Source: CAD feature listing. Evaluate the final solid. Frame: model axes, mm. A direction names the side the tool comes from. Round coordinates to 2 decimals unless told otherwise and drop trailing zeros. Write each loop counter-clockwise with the first axis right and the second up, starting at its lowest first coordinate (ties: lowest second). Pieces come first, ordered by that corner, then holes. Notation, with made-up numbers: M 17,-17.5 L 29,-17.5 A5 cw 29,-12.5 Z; hole C 42,43 d8. An arc over 180 degrees is marked long. Answer in a Markdown table with one row per item. Add a question column.
Item 1: Mould query, pull axis Z, two halves, no side actions, for faces 1 (the face through (84.3, -5, 0)), 2 (the face through (94, 2, -10)), 3 (the face through (92.6, 0.1, 9)). Classes: released by +Z, released by -Z, zero draft, split by the parting line, or undercut.
Item 2: Material intervals for probe 1 along Z at (x, y) = (2, -1.1); probe 2 along Y at (x, z) = (95, -9.55); probe 3 along X at (y, z) = (1.3, 0), sorted ascending.
Item 3: Contact query for flat-ended pins moving along their axis: pin 1 (1.5 mm diameter, centred on y = 2, z = 0.5, fed in from +X); pin 2 (0.6 mm diameter, centred on y = -0.5, z = 0, fed in from -X); pin 3 (1.8 mm diameter, centred on x = 2.5, z = 0, fed in from +Y). Output: stop coordinate, or through.
Item 4: Set-up query: faces 4 (the face through (41.41, -1.5, -0.07)), 5 (the face through (2.5, -1, -0.5)), 6 (the face through (85, 0, 0)). Return all of +Z, -Z, +X, -X, +Y, -Y with unobstructed straight access to the full face (end or side cutting, diameter ignored); none if empty.
Item 5: Cut plane B-B on y = 0. Return loops of the section in (x, z).
Item 6: Cut plane A-A on x = 95. Return loops of the section in (y, z), and give its area (3 significant figures).
Item 7: Cut plane C-C on z = 8. Return loops of the section in (x, y).
Item 8: Cut plane D-D on x = 50. Return loops of the section in (y, z).
Autodesk Inventor part; units mm, degrees
ref_plane "YZ Plane" through (0, 0, 0) normal (1, 0, 0) x (0, 1, 0)
ref_plane "XZ Plane" through (0, 0, 0) normal (0, 1, 0) x (-1, 0, 0)
ref_plane "XY Plane" through (0, 0, 0) normal (0, 0, 1) x (1, 0, 0)
sketch "草图1" plane through (0, 0, 0) normal (1, 0, 0) x (0, 1, 0)
  circle A0 centre (0, 0) radius 1.5
  dimension "杆直径" = 3
extrude "拉伸1" add sketch "草图1" along normal blind 84
sketch "草图2" plane through (84, 0, 0) normal (1, 0, 0) x (0, 0, -1)
  line L0 (10, -5) -> (-10, -5)
  line L1 (-10, -5) -> (-10, 5)
  line L2 (-10, 5) -> (10, 5)
  line L3 (10, 5) -> (10, -5)
  line L4 (10, -5) -> (-10, 5) construction
  line L5 (-10, -5) -> (10, 5) construction
  point P0 (0, 0)
  dimension "框长" = 20
  dimension "框宽" = 10
extrude "拉伸2" add sketch "草图2" along normal blind 1
sketch "草图3" plane through (85, 0, 0) normal (1, 0, 0) x (0, 0, -1)
  line L0 (-10, -5) -> (10, -5)
  line L1 (10, -5) -> (10, 5)
  line L2 (10, 5) -> (-10, 5)
  line L3 (-10, 5) -> (-10, -5)
  line L4 (-10, 5) -> (-9, 5)
  line L5 (-9, 5) -> (-9, -5)
  line L6 (10, 5) -> (9, 5)
  line L7 (9, 5) -> (9, -5)
  point P0 (0, 0)
  dimension "d7" = 1
  dimension "d8" = 1
extrude "拉伸3" add sketch "草图3" along normal blind 20 contours L3 L2 L5 L0 | L7 L2 L1 L0
hole "孔1" at (95, 0, -10) direction (0, 0, 1) diameter 4 end through all
sketch "草图5" plane through (0, 0, 0) normal (0, 0, 1) x (1, 0, 0)
  line L0 (0, 1.5) -> (0, -1.5)
  line L1 (0, 1.5) -> (84, 1.5)
  line L2 (0, -1.5) -> (84, -1.5)
  line L3 (0, 1) -> (4, 1)
  line L4 (4, 1) -> (4, -1)
  line L5 (4, -1) -> (0, -1)
  line L6 (0, 0) -> (4, 0) construction
  point P0 (2, 0)
  dimension "d21" = 4
  dimension "宽度" = 2
extrude "拉伸4" cut sketch "草图5" along normal through all both and the other way through all
sketch "草图6" plane through (0, 0, 0) normal (0, 1, 0) x (-1, 0, 0)
  line L0 (-4, 1.5) -> (-84, 1.5)
  line L1 (-4, -1.5) -> (-84, -1.5)
  line L2 (0, 1.118) -> (0, -1.118)
  line L3 (-4, -1.118) -> (-4, 1.118)
  circle A0 centre (-2, 0) radius 0.5
  point P0 (0, 0)
  dimension "位置1" = 2
  dimension "位置2" = 1.5
  dimension "销孔径" = 1
extrude "拉伸5" cut sketch "草图6" along normal mid plane 10
properties part number "顶杆" material "木材(桦木)"
Results below:
| question | item | result |
|---|---|---|
| 1 | face 1 | zero draft |
| 1 | face 2 | released by -Z |
| 1 | face 3 | undercut |
| 2 | probe 1 | -1.02 to -0.5, 0.5 to 1.02 |
| 2 | probe 2 | -5 to -2, 2 to 5 |
| 2 | probe 3 | 0 to 1.5, 2.5 to 85 |
| 3 | pin 1 | x = 85 |
| 3 | pin 2 | x = 4 |
| 3 | pin 3 | y = 1.5 |
| 4 | face 4 | -X |
| 4 | face 5 | +Z, -Z, -X |
| 4 | face 6 | +X, +Y, -Y |
| 5 | outline | M 4,-1.5 L 84,-1.5 L 84,-10 L 93,-10 L 93,-9 L 85,-9 L 85,9 L 93,9 L 93,10 L 84,10 L 84,1.5 L 4,1.5 Z; M 97,-10 L 105,-10 L 105,-9 L 97,-9 Z; M 97,9 L 105,9 L 105,10 L 97,10 Z |
| 6 | outline | M -5,-10 L -2,-10 L -2,-9 L -5,-9 Z; M -5,9 L -2,9 L -2,10 L -5,10 Z; M 2,-10 L 5,-10 L 5,-9 L 2,-9 Z; M 2,9 L 5,9 L 5,10 L 2,10 Z |
| 6 | area | 12.0 mm2 |
| 7 | outline | M 84,-5 L 85,-5 L 85,5 L 84,5 Z |
| 8 | outline | C 0,0 d3 |
